Could you check a few things on this model? Use its own coordinates, in mm. A direction names the side the tool comes from. Give positions to 0.01 mm unless a question says otherwise; leave off trailing zeros. Write each loop counter-clockwise with the first axis right and the second up, starting at its lowest first coordinate (ties: lowest second). Pieces come first, ordered by that corner, then holes. Notation, with made-up numbers: (-39, 24) - (20, 24) arc R12 ccw to (20, 42) - close; hole circle Ø5 at (49.5, -4.75). An arc over 180 degrees is marked (long way). Write item = value, one per line.
from build123d import *

# Parameters (mm, degrees)
F0_W      = 96
F0_H      = 64
F1_DEPTH  = 16
F3_DEPTH  = 16.001
F4_W      = 16
F4_H      = 64
F5_DEPTH  = 48
F6_R      = 32
F7_W      = 40
F7_H      = 42
F8_DEPTH  = 28
F10_DEPTH = 42.001
F12_DEPTH = 12
F13_R     = 3.560892
F14_DEPTH = 64.001


with BuildPart() as f1:
    # F0 (on Top) → F1 (new body)
    with BuildSketch(Plane.XY):
        with Locations((48, 32)):
            Rectangle(F0_W, F0_H)
    extrude(amount=F1_DEPTH)

    # F2 (on face) → F3 (cut, through all)
    with BuildSketch(Plane.XY.offset(16)):
        with BuildLine():
            ThreePointArc((76, 32), (68, 24), (76, 16))
            Line((76, 16), (96, 16))
            Line((96, 16), (96, 32))
            Line((96, 32), (76, 32))
        make_face()
    extrude(amount=-F3_DEPTH, mode=Mode.SUBTRACT)

    # F4 (on face) → F5 (join)
    with BuildSketch(Plane.XY.offset(16)):
        with Locations((8, 32)):
            Rectangle(F4_W, F4_H)
    extrude(amount=F5_DEPTH)

    # F6
    f6_edges = [f1.edges().sort_by_distance(p)[0] for p in [
        (8, 0, 64),
    ]]
    fillet(f6_edges, radius=F6_R)

    # F7 (on face) → F8 (join)
    with BuildSketch(Plane.XY.offset(16)):
        with Locations((36, 43)):
            Rectangle(F7_W, F7_H)
    extrude(amount=F8_DEPTH)

    # F9 (on face) → F10 (cut, through all)
    with BuildSketch(Plane.XZ.offset(-22)):
        with BuildLine():
            ThreePointArc((24, 44), (36, 32), (48, 44))
            Line((48, 44), (24, 44))
        make_face()
        with BuildLine():
            Line((24, 44), (48, 44))
            ThreePointArc((48, 44), (36, 56), (24, 44))
        make_face()
    extrude(amount=-F10_DEPTH, mode=Mode.SUBTRACT)

    # F11 (on face) → F12 (join)
    with BuildSketch(Plane(origin=(0, 64, 0), x_dir=(-1, 0, 0), z_dir=(0, 1, 0))):
        Polygon((-56, 16), (-56, 44), (-96, 16), align=None)
    extrude(amount=-F12_DEPTH)

    # F13 (on face) → F14 (cut, through all)
    with BuildSketch(Plane.XZ):
        with Locations((41.068658, 6.811937)):
            Circle(F13_R)
    extrude(amount=-F14_DEPTH, mode=Mode.SUBTRACT)


solid = f1.part
1. Thinking about a two-plate mould opening in X: for faces 1 (the face through (0, 32, 32)), 2 (the face through (64, 21, 16)), 3 (the face through (36, 43, 32)), 4 (the face through (96, 48, 8)), which applies, pulls with the +X half, pulls with the -X half, needs draft (parallel to the pull), parting line crosses it, or undercut?
Filled sheet:
face_1 = pulls with the -X half
face_2 = needs draft
face_3 = undercut
face_4 = pulls with the +X half
2. If we section it at B-B, the plane z = 37: Please give me the cut outline in (x, y), and give its area (3 significant figures).
Filled sheet:
outline = (0, 0.39) - (16, 0.39) - (16, 22) - (26.25, 22) - (26.25, 64) - (0, 64) - close; (45.75, 22) - (56, 22) - (56, 52) - (66, 52) - (66, 64) - (45.75, 64) - close
area = 2,000 mm2
3. Which directions (+Z, -Z, +X, -X, +Y, -Y) give clear straight access to the entire face, cutting with the end or side of a thin tool? Please do faces 5 (the face through (37, 0, 12)), 6 (the face through (67, 52, 24)), 7 (the face through (20, 43, 44)), 8 (the face through (86, 16, 8)).
Filled sheet:
face_5 = +Z, -Z, +X, -X, -Y
face_6 = +Z, +X, -Y
face_7 = +Z, +X, +Y, -Y
face_8 = +Z, -Z, +X
4. For pin 1 (6 mm diameter, centred on x = 77.5, z = 20.5, fed in from -Y); pin 2 (12 mm diameter, centred on x = 46.5, y = 40, fed in from +Z); pin 3 (24 mm diameter, centred on y = 24, z = 39.5, fed in from +X), each with a flat end and sliding along its axis, tell me the tip position at first contact or that it passes through.
Filled sheet:
pin_1 = 52
pin_2 = 44
pin_3 = 56
5. I need wall thicknesses on line 1 (X direction, y = 24, z = 7); line 2 (X direction, y = 46.5, z = 6.5); line 3 (X direction, y = 49.5, z = 60.5). Which ranges of each line are inside material? Lowest first, please.
Filled sheet:
line_1 = 0 to 37.51, 44.62 to 68
line_2 = 0 to 37.52, 44.62 to 96
line_3 = 0 to 16
6. If we section it at C-C, the plane y = 20.5: Please give me the cut outline in (x, z).
Filled sheet:
outline = (0, 0) - (68.81, 0) - (68.81, 16) - (16, 16) - (16, 61.86) - (0, 61.86) - close; hole circle Ø7.12 at (41.07, 6.81)
7. If we section it at A-A, the plane x = 85.5: Please give me the cut outline in (y, z).
Filled sheet:
outline = (0, 0) - (16, 0) - (16, 16) - (0, 16) - close; (32, 0) - (64, 0) - (64, 23.35) - (52, 23.35) - (52, 16) - (32, 16) - close
8. If we section it at D-D, the plane x = 40.5: Please give me the cut outline in (y, z), and give its area (3 significant figures).
Filled sheet:
outline = (0, 0) - (64, 0) - (64, 3.3) - (0, 3.3) - close; (0, 10.33) - (64, 10.33) - (64, 32.88) - (22, 32.88) - (22, 16) - (0, 16) - close
area = 1,280 mm2
